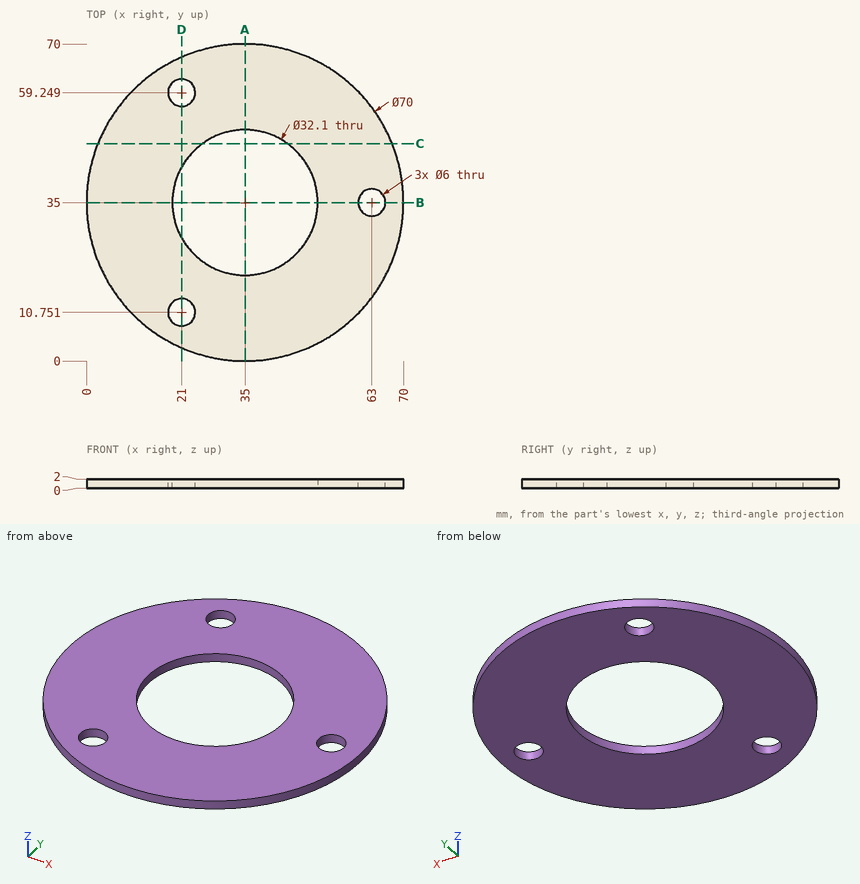
Study the drawing (mm; zero at the part's minimum x, y, z) and answer. Coordinates: 2 decimals unless noted, no trailing zeros. Write each loop counter-clockwise with the first axis right and the second up, starting at its lowest first coordinate (ties: lowest second). Pieces come first, ordered by that corner, then holes. Notation, with made-up numbers: (8.5, 76.25) - (14.5, 76.25) arc R19 ccw to (14.5, 112.25) - close; hole circle Ø9 at (86.25, -35.5). An arc over 180 degrees is marked (long way). Put each result on its own line as item: value.
1. Flat-ended cylindrical pins translate along their axes: pin 1 Ø8 at (x, y) = (25.5, 35) entering from +Z; pin 2 Ø1 at (y, z) = (26, 2) entering from +X. Find the tip coordinate at first contact, or state that the pin passes through.
Answer sheet:
pin 1: passes through
pin 2: stops at x = 68.95
2. The part is cut by section C-C on y = 48. Give the vertices of the cut face in (x, z).
Answer sheet:
outline: (2.5, 0) - (25.59, 0) - (25.59, 2) - (2.5, 2) - close; (44.41, 0) - (67.5, 0) - (67.5, 2) - (44.41, 2) - close
3. Find the intervals of material crossed by line 1 along Y through (x, z) = (34.5, 0.55); line 2 along Y through (x, z) = (22, 1.45) (1 decimal); line 3 along X through (y, z) = (10.5, 0.7) (1 decimal), in increasing order. Write a range as from..to.
Answer sheet:
line 1: y = 0..18.96, 51.04..70
line 2: y = 2.5..7.9, 13.6..25.6, 44.4..56.4, 62.1..67.5
line 3: x = 10..18, 24..60
4. The part is cut by section D-D on x = 21. Give the vertices of the cut face in (y, z).
Answer sheet:
outline: (2.92, 0) - (7.75, 0) - (7.75, 2) - (2.92, 2) - close; (13.75, 0) - (27.15, 0) - (27.15, 2) - (13.75, 2) - close; (42.85, 0) - (56.25, 0) - (56.25, 2) - (42.85, 2) - close; (62.25, 0) - (67.08, 0) - (67.08, 2) - (62.25, 2) - close
5. The part is cut by section A-A on x = 35. Give the vertices of the cut face in (y, z), plus the area to 3 significant figures.
Answer sheet:
outline: (0, 0) - (18.95, 0) - (18.95, 2) - (0, 2) - close; (51.05, 0) - (70, 0) - (70, 2) - (51.05, 2) - close
area: 75.8 mm^2
6. The part is cut by section B-B on y = 35. Give the vertices of the cut face in (x, z).
Answer sheet:
outline: (0, 0) - (18.95, 0) - (18.95, 2) - (0, 2) - close; (51.05, 0) - (60, 0) - (60, 2) - (51.05, 2) - close; (66, 0) - (70, 0) - (70, 2) - (66, 2) - close
